CAD build for the part. Positions are in the model's coordinates, mm. Coordinates: 2 decimals unless noted, no trailing zeros. Order: outer loops, then holes, each group sorted by start corner. A loop starts at its lowest first (then second) coordinate and runs counter-clockwise, first axis right, second up. Notation, with made-up numbers: M -6.75,-11.5 L 27.25,-11.5 A9 ccw 27.25,-5.5 Z; hole C 77,38 d8. An arc over 180 degrees is marked long. Write item = value, one per line. Start each with the question number.
```python
from build123d import *

# Parameters (mm, degrees)
BOSS_EXTRUDE1_DEPTH = 6
SKETCH2_R           = 12.2
BOSS_EXTRUDE2_DEPTH = 5.25


with BuildPart() as part:
    # Sketch1 → Boss-Extrude1 (new body)
    with BuildSketch(Plane.XY):
        with BuildLine():
            Line((53.452478751, 19.630204959), (303.423888155, 15.84917852))
            ThreePointArc((303.423888155, 15.84917852), (323.119118527, -4.451016075), (302.818923933, -24.146246447))
            Line((302.818923933, -24.146246447), (52.847514529, -20.365220008))
            ThreePointArc((52.847514529, -20.365220008), (33.152284157, -0.065025413), (53.452478751, 19.630204959))
        make_face()
    extrude(amount=BOSS_EXTRUDE1_DEPTH)

    # Sketch2 → Boss-Extrude2 (add)
    with BuildSketch(Plane(origin=(0, 0, 0), x_dir=(-1, 0, 0), z_dir=(0, 0, -1))):
        with Locations((-53.14999664, -0.367507524)):
            Circle(SKETCH2_R)
    extrude(amount=BOSS_EXTRUDE2_DEPTH)


solid = part.part
```
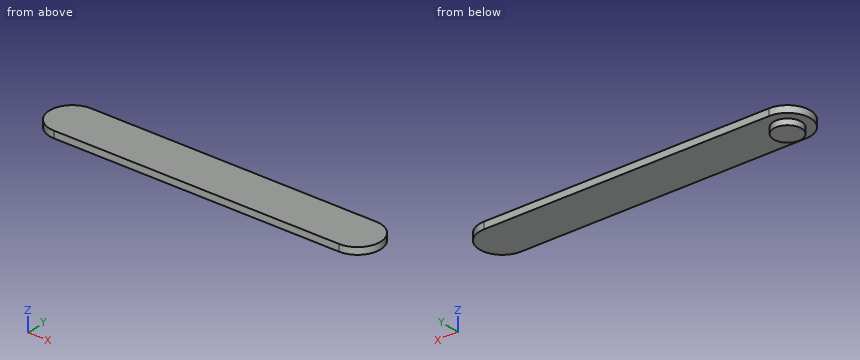
1. Probe L1, parallel to Z at x = 288, y = -13; L2, parallel to Y at x = 164, z = 4.75; L3, parallel to X at y = -9, z = -0.75. List the from-to ranges inside material, lowest first.
2. Slice it at A-A (z = 3). Write the cut outline in (x, y).
3. Flat gauge pins, fed straight in: pin 1 (2 mm diameter, centred on x = 67.5, y = 1.5, fed in from -Z); pin 2 (1 mm diameter, centred on x = 172.5, z = 3.5, fed in from -Y); pin 3 (6 mm diameter, centred on y = -7.5, z = -0.5, fed in from +X). Where does each tip first touch, or does it go through?
4. Slice it at B-B (x = 282). Write the cut outline in (y, z).
Calculated:
q1.L1 = 0 to 6
q1.L2 = -22.05 to 17.96
q1.L3 = 44.53 to 61.77
q2.outline = M 52.85,-20.37 L 302.82,-24.15 A20 ccw 303.42,15.85 L 53.45,19.63 A20 ccw Z
q3.pin_1 = 0
q3.pin_2 = -22.18
q3.pin_3 = 323.12
q4.outline = M -23.83,0 L 16.17,0 L 16.17,6 L -23.83,6 Z
